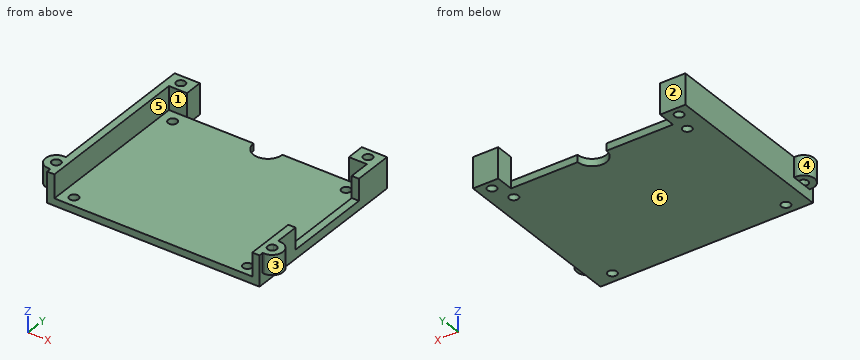
from build123d import *
from build123d.topology import SkipClean

# Parameters (mm, degrees)
BOSS_EXTRUDE1_DEPTH = 44.5
SKETCH2_W           = 6
SKETCH2_H           = 24.6
CUT_EXTRUDE1_DEPTH  = 10
BOSS_EXTRUDE2_DEPTH = 8.5
CUT_EXTRUDE2_DEPTH  = 11
SKETCH4_W           = 7
SKETCH4_H           = 8.5
BOSS_EXTRUDE3_DEPTH = 5
SKETCH5_R           = 1.25
CUT_EXTRUDE3_DEPTH  = 81.179486155
SKETCH7_R           = 1.25
CUT_EXTRUDE4_DEPTH  = 10
SKETCH8_R           = 4
CUT_EXTRUDE5_DEPTH  = 81.179486155
CUT_EXTRUDE6_DEPTH  = 3
BOSS_EXTRUDE4_DEPTH = 3


with BuildPart() as part:
    # Sketch1 → Boss-Extrude1 (new body)
    with BuildSketch(Plane(origin=(0, 0, 0), x_dir=(1, 0, 0), z_dir=(0, 1, 0))):
        Polygon((0, 0), (2, 0), (2, 6.5), (57, 6.5), (57, 0), (59, 0), (59, 8.5), (0, 8.5), align=None)
    extrude(amount=BOSS_EXTRUDE1_DEPTH)

    # Sketch2 → Cut-Extrude1 (cut)
    with BuildSketch(Plane(origin=(59, 0, 0), x_dir=(0, 0, -1), z_dir=(1, 0, 0))):
        with Locations((3, 26.3)):
            Rectangle(SKETCH2_W, SKETCH2_H)
    extrude(amount=-CUT_EXTRUDE1_DEPTH, mode=Mode.SUBTRACT)

    # Sketch3 → Boss-Extrude2 (add)
    with BuildSketch(Plane(origin=(0, 0, -8.5), x_dir=(-1, 0, 0), z_dir=(0, 0, -1))):
        with BuildLine():
            Line((-59, 5.395643924), (-59, 7.25))
            Line((-59, 7.25), (-59.5, 7.25))
            ThreePointArc((-59.5, 7.25), (-62.5, 4.25), (-59.5, 1.25))
            Line((-59.5, 1.25), (-59, 1.25))
            Line((-59, 1.25), (-59, 3.104356076))
            ThreePointArc((-59, 3.104356076), (-60.75, 4.25), (-59, 5.395643924))
        make_face()
        with BuildLine():
            Line((0.5, 7.25), (0, 7.25))
            Line((0, 7.25), (0, 5.395643924))
            ThreePointArc((0, 5.395643924), (1.184653197, 5.295825033), (1.75, 4.25))
            ThreePointArc((1.75, 4.25), (1.184653197, 3.204174967), (0, 3.104356076))
            Line((0, 3.104356076), (0, 1.25))
            Line((0, 1.25), (0.5, 1.25))
            ThreePointArc((0.5, 1.25), (3.5, 4.25), (0.5, 7.25))
        make_face()
    extrude(amount=-BOSS_EXTRUDE2_DEPTH)

    # Sketch3_3 → Cut-Extrude2 (cut)
    with SkipClean():  # the faces are left unmerged after this step: merging them gives an invalid solid
        with BuildSketch(Plane(origin=(0, 0, -8.5), x_dir=(-1, 0, 0), z_dir=(0, 0, -1))):
            with BuildLine():
                ThreePointArc((-58.25, 4.25), (-58.454174967, 4.934653197), (-59, 5.395643924))
                Line((-59, 5.395643924), (-59, 3.104356076))
                ThreePointArc((-59, 3.104356076), (-58.454174967, 3.565346803), (-58.25, 4.25))
            make_face()
            with BuildLine():
                Line((-59, 3.104356076), (-59, 5.395643924))
                ThreePointArc((-59, 5.395643924), (-60.75, 4.25), (-59, 3.104356076))
            make_face()
            with BuildLine():
                ThreePointArc((1.75, 4.25), (1.184653197, 5.295825033), (0, 5.395643924))
                Line((0, 5.395643924), (0, 3.104356076))
                ThreePointArc((0, 3.104356076), (1.184653197, 3.204174967), (1.75, 4.25))
            make_face()
            with BuildLine():
                Line((0, 3.104356076), (0, 5.395643924))
                ThreePointArc((0, 5.395643924), (-0.75, 4.25), (0, 3.104356076))
            make_face()
        extrude(amount=-CUT_EXTRUDE2_DEPTH, mode=Mode.SUBTRACT)

    # Sketch4 → Boss-Extrude3 (add)
    with SkipClean():  # the faces are left unmerged after this step: merging them gives an invalid solid
        with BuildSketch(Plane(origin=(0, 44.5, 0), x_dir=(1, 0, 0), z_dir=(0, 1, 0))):
            with Locations((3.5, 4.25)):
                Rectangle(SKETCH4_W, SKETCH4_H)
            with Locations((55.5, 4.25)):
                Rectangle(SKETCH4_W, SKETCH4_H)
        extrude(amount=BOSS_EXTRUDE3_DEPTH)

    # Sketch5 → Cut-Extrude3 (cut, through all)
    with SkipClean():  # the faces are left unmerged after this step: merging them gives an invalid solid
        with BuildSketch(Plane(origin=(0, 0, -8.5), x_dir=(-1, 0, 0), z_dir=(0, 0, -1))):
            with Locations((-55.5, 47)):
                Circle(SKETCH5_R)
            with Locations((-3.5, 47)):
                Circle(SKETCH5_R)
        extrude(amount=-CUT_EXTRUDE3_DEPTH, mode=Mode.SUBTRACT)

    # Sketch7 → Cut-Extrude4 (cut)
    with SkipClean():  # the faces are left unmerged after this step: merging them gives an invalid solid
        with BuildSketch(Plane(origin=(0, 0, -8.5), x_dir=(-1, 0, 0), z_dir=(0, 0, -1))):
            with Locations((-53.6, 2.9)):
                Circle(SKETCH7_R)
            with Locations((-5.4, 2.9)):
                Circle(SKETCH7_R)
            with Locations((-53.6, 41.2)):
                Circle(SKETCH7_R)
            with Locations((-5.4, 41.2)):
                Circle(SKETCH7_R)
        extrude(amount=-CUT_EXTRUDE4_DEPTH, mode=Mode.SUBTRACT)

    # Sketch8 → Cut-Extrude5 (cut, through all)
    with SkipClean():  # the faces are left unmerged after this step: merging them gives an invalid solid
        with BuildSketch(Plane(origin=(0, 0, -8.5), x_dir=(-1, 0, 0), z_dir=(0, 0, -1))):
            with Locations((-29.5, 44.5)):
                Circle(SKETCH8_R)
        extrude(amount=-CUT_EXTRUDE5_DEPTH, mode=Mode.SUBTRACT)

    # Sketch3_4 → Cut-Extrude6 (cut)
    with SkipClean():  # the faces are left unmerged after this step: merging them gives an invalid solid
        with BuildSketch(Plane(origin=(0, 0, -8.5), x_dir=(-1, 0, 0), z_dir=(0, 0, -1))):
            with BuildLine():
                Line((-59, 5.395643924), (-59, 7.25))
                Line((-59, 7.25), (-59.5, 7.25))
                ThreePointArc((-59.5, 7.25), (-62.5, 4.25), (-59.5, 1.25))
                Line((-59.5, 1.25), (-59, 1.25))
                Line((-59, 1.25), (-59, 3.104356076))
                ThreePointArc((-59, 3.104356076), (-60.75, 4.25), (-59, 5.395643924))
            make_face()
            with BuildLine():
                Line((0.5, 7.25), (0, 7.25))
                Line((0, 7.25), (0, 5.395643924))
                ThreePointArc((0, 5.395643924), (1.184653197, 5.295825033), (1.75, 4.25))
                ThreePointArc((1.75, 4.25), (1.184653197, 3.204174967), (0, 3.104356076))
                Line((0, 3.104356076), (0, 1.25))
                Line((0, 1.25), (0.5, 1.25))
                ThreePointArc((0.5, 1.25), (3.5, 4.25), (0.5, 7.25))
            make_face()
        extrude(amount=-CUT_EXTRUDE6_DEPTH, mode=Mode.SUBTRACT)

    # Sketch3_5 → Boss-Extrude4 (add)
    with SkipClean():  # the faces are left unmerged after this step: merging them gives an invalid solid
        with BuildSketch(Plane(origin=(0, 0, -8.5), x_dir=(-1, 0, 0), z_dir=(0, 0, -1))):
            with BuildLine():
                ThreePointArc((-59, 3.104356076), (-58.25, 4.25), (-59, 5.395643924))
                Line((-59, 5.395643924), (-59, 3.104356076))
            make_face()
            with BuildLine():
                Line((0, 3.104356076), (0, 5.395643924))
                ThreePointArc((0, 5.395643924), (-0.75, 4.25), (0, 3.104356076))
            make_face()
        extrude(amount=-BOSS_EXTRUDE4_DEPTH)


solid = part.part
Work out the finished part from the listing and answer in its coordinate system (mm). Face numbers are marked on the shaded views. A direction names the side the tool comes from. Coordinates: 2 decimals unless noted, no trailing zeros. Write each loop counter-clockwise with the first axis right and the second up, starting at its lowest first coordinate (ties: lowest second). Pieces come first, ordered by that corner, then holes. Notation, with made-up numbers: M -14,44 L 6,44 A31 ccw 6,72 Z; hole C 30,-9 d6. An arc over 180 degrees is marked long. Use one line per item in the form item = value. Start each with the question number.
1. The mould has two halves that part along X. Classify the marked faces 1, 2, 3 and 4: released by +X, released by -X, zero draft, split by the parting line, or undercut.
2. A tool of negligible diameter and unlimited length cuts with its end or side. For the marked faces 5 and 6, from which of +Z, -Z, +X, -X, +Y, -Y can it reach the whole face along a straight path? Write none if from no direction.
3. The part is cut by section A-A (y = 47). Give the vertices of the cut face in (x, z), plus the area to 3 significant figures.
4. The part is cut by section C-C (y = 16). Give the vertices of the cut face in (x, z).
5. Each of these flat-tipped pins is pushed along its axis until it touches: P1, Ø3, axis at x = 61, y = 3, coming from the -Z side; P2, Ø0.6, axis at x = 58.5, y = 27, coming from the +Z side; P3, Ø1.5, axis at y = 37, z = -3, coming from the -X side. Where does it stop, or does it pass through?
6. The part is cut by section D-D (x = 38.5). Give the vertices of the cut face in (y, z).
7. Straight lines are drawn through the part: probe 1 along Y at (x, z) = (5.4, -7.35); probe 2 along X at (y, z) = (39, -4.5); probe 3 along X at (y, z) = (4.5, -4). For each, find the intervals that lie inside material, in ascending order. Write a range as from..to.
8. The part is cut by section B-B (z = -7.5). Give the vertices of the cut face in (x, y).
Evaluation:
q1.face_1 = undercut
q1.face_2 = zero draft
q1.face_3 = released by +X
q1.face_4 = released by -X
q2.face_5 = +Z, -Y
q2.face_6 = -Z, +X, -X, +Y, -Y
q3.outline = M 0,-8.5 L 2.25,-8.5 L 2.25,0 L 0,0 Z; M 4.75,-8.5 L 7,-8.5 L 7,0 L 4.75,0 Z; M 52,-8.5 L 54.25,-8.5 L 54.25,0 L 52,0 Z; M 56.75,-8.5 L 59,-8.5 L 59,0 L 56.75,0 Z
q3.area = 76.5 mm^2
q4.outline = M 0,-8.5 L 59,-8.5 L 59,-6 L 57,-6 L 57,-6.5 L 2,-6.5 L 2,0 L 0,0 Z
q5.P1 = -5.5
q5.P2 = -6
q5.P3 = 0
q6.outline = M 0,-8.5 L 44.5,-8.5 L 44.5,-6.5 L 0,-6.5 Z
q7.probe_1 = 0..1.65, 4.15..39.95, 42.45..49.5
q7.probe_2 = 0..2, 57..59
q7.probe_3 = -3.49..-1.72, 0.72..2, 57..58.28, 60.72..62.49
q8.outline = M 0,0 L 59,0 L 59,49.5 L 52,49.5 L 52,44.5 L 33.5,44.5 A4 cw 25.5,44.5 L 7,44.5 L 7,49.5 L 0,49.5 Z; hole C 3.5,47 d2.5; hole C 5.4,2.9 d2.5; hole C 5.4,41.2 d2.5; hole C 53.6,2.9 d2.5; hole C 53.6,41.2 d2.5; hole C 55.5,47 d2.5
